Answer from the drawing. Dimensions are ordinates in mm from the lowest x, y and z of the part. A direction names the side the tool comes from. Give positions to 0.01 mm unless a question says otherwise; leave off trailing zeros. Loops run counter-clockwise (first coordinate to the right, second up) from the corner with the lowest first, then second, coordinate; pieces in that order, holes last. Notation, with made-up numbers: (75, -35.5) - (99, -35.5) arc R18 ccw to (99, -9.5) - close; hole circle Ø8 at (-27, 88). An arc over 180 degrees is marked (long way). Write each question's results on one line, items separated by ' | '. Start each with the question number.
Q1. The part is cut by section D-D, the plane y = 22. Write down the section's boundary in (x, z).
Q2. The part is cut by section B-B, the plane x = 42.5. Write down the section's boundary in (y, z).
Q3. Find the intervals of material crossed by line 1 (Y direction, x = 42.5, z = 9.5); line 2 (Y direction, x = 41, z = 7); line 3 (Z direction, x = 80, y = 26), in increasing order. Write a range as from..to.
Q4. For the marked faces 1 and 2, determine the directions among +Z, -Z, +X, -X, +Y, -Y from which every point of the face is accessible in a straight line to the end or side of a thin tool.
Q5. Determine the mould class of the marked faces 3, 4 and 5 for opening direction Y: +Y half, -Y half, draft (parallel to the pull), parting line (faces both ways), or undercut.
Q6. Given pin 1 (1 mm diameter, centred on x = 33, z = 4.5, fed in from +Y); pin 2 (4 mm diameter, centred on y = 15, z = 9.5, fed in from +X); pin 3 (8 mm diameter, centred on x = 36, z = 7.5, fed in from +Y), each flat-ended and moving along its own axis, determine where each tip first touches the part or whether it passes through.
Q7. The part is cut by section C-C, the plane z = 9.25. Write down the section's boundary in (x, y).
Q8. The part is cut by section A-A, the plane y = 42.5. Write down the section's boundary in (x, z).
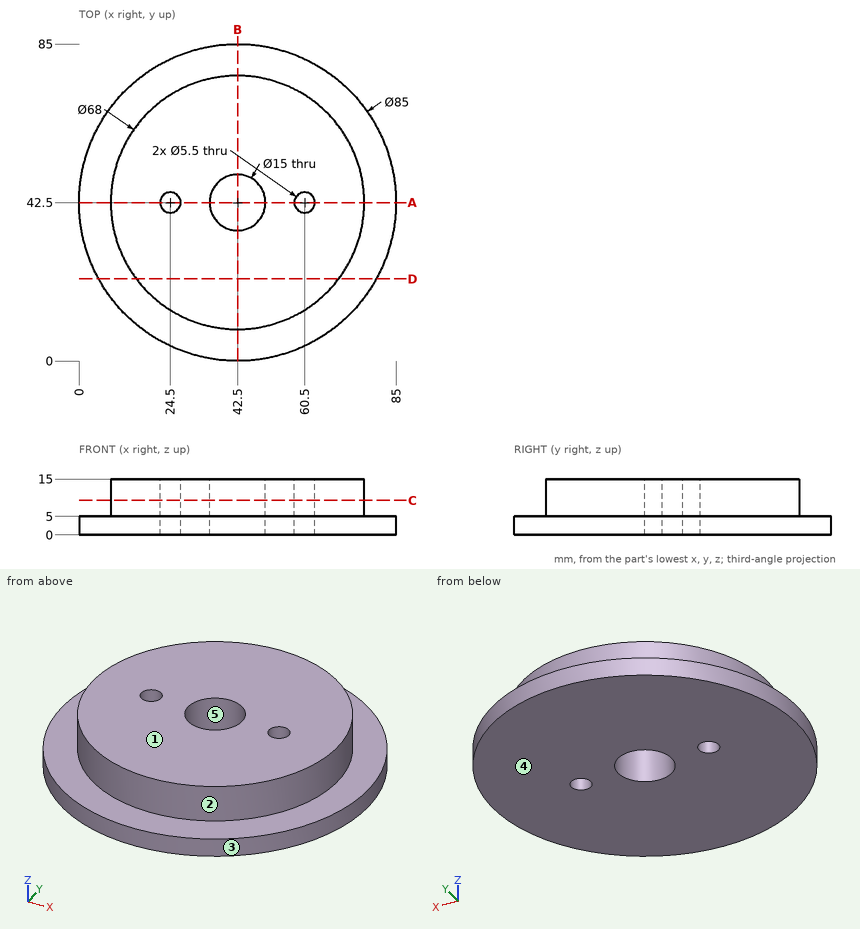
Check sheet entries:
1) outline: (5.27, 0) - (79.73, 0) - (79.73, 5) - (69.62, 5) - (69.62, 15) - (15.38, 15) - (15.38, 5) - (5.27, 5) - close
2) outline: (0, 0) - (35, 0) - (35, 15) - (8.5, 15) - (8.5, 5) - (0, 5) - close; (50, 0) - (85, 0) - (85, 5) - (76.5, 5) - (76.5, 15) - (50, 15) - close
3) line 1: y = 8.5..35, 50..76.5 | line 2: y = 8.53..35.15, 49.85..76.47 | line 3: z = 0..5
4) face 1: +Z, +X, -X, +Y, -Y | face 2: +Z
5) face 3: parting line | face 4: draft | face 5: undercut
6) pin 1: stops at y = 84.04 | pin 2: stops at x = 64.99 | pin 3: stops at y = 84.87
7) outline: circle Ø68 at (42.5, 42.5); hole circle Ø5.5 at (24.5, 42.5); hole circle Ø15 at (42.5, 42.5); hole circle Ø5.5 at (60.5, 42.5)
8) outline: (0, 0) - (21.75, 0) - (21.75, 15) - (8.5, 15) - (8.5, 5) - (0, 5) - close; (27.25, 0) - (35, 0) - (35, 15) - (27.25, 15) - close; (50, 0) - (57.75, 0) - (57.75, 15) - (50, 15) - close; (63.25, 0) - (85, 0) - (85, 5) - (76.5, 5) - (76.5, 15) - (63.25, 15) - close
